The model under review builds one solid part; all positions refer to its coordinate system, in mm. A direction names the side the tool comes from. Give positions to 0.01 mm unless a question says otherwise; leave off trailing zeros. Order: outer loops, then holes, each group sorted by start corner. A loop starts at its lowest first (then second) coordinate and runs counter-clockwise, first axis right, second up. Notation, with made-up numbers: (-36, -13.5) - (8, -13.5) arc R25 cw to (8, -1.5) - close; hole circle Ø5 at (58.5, 82). An arc over 180 degrees is marked (long way). Use a Markdown table: item, result. Add a question column.
```python
from build123d import *

# Parameters (mm, degrees)
SKETCH2_R               = 1.651
BOSS_EXTRUDE1_DEPTH     = 68.58
CUT_EXTRUDE3_DEPTH      = 79.441187854
CUT_EXTRUDE3_DEPTH_BACK = 79.441187854
SKETCH3_R               = 3


with BuildPart() as part:
    # Sketch2 → Boss-Extrude1 (new body)
    with BuildSketch(Plane(origin=(0, 0, 0), x_dir=(0, 0, -1), z_dir=(1, 0, 0))):
        with BuildLine():
            Line((-12.7, 12.7), (12.7, 12.7))
            Line((12.7, 12.7), (12.7, 0))
            Line((12.7, 0), (26.924, 0))
            ThreePointArc((26.924, 0), (0, 26.924), (-26.924, 0))
            Line((-26.924, 0), (-12.7, 0))
            Line((-12.7, 0), (-12.7, 12.7))
        make_face()
        with Locations((14.368409794, 14.368409794)):
            Circle(SKETCH2_R, mode=Mode.SUBTRACT)
        with Locations((-14.368409794, 14.368409794)):
            Circle(SKETCH2_R, mode=Mode.SUBTRACT)
    extrude(amount=BOSS_EXTRUDE1_DEPTH)

    # Sketch3 → Cut-Extrude3 (cut, two sides: drawn at the far end of the back side and taken through both)
    with BuildSketch(Plane(origin=(0, 0, 0), x_dir=(1, 0, 0), z_dir=(0, 1, 0)).offset(-CUT_EXTRUDE3_DEPTH_BACK)):
        with Locations(Location((34.57387325, 0, 0), (0, 0, 180))):
            Circle(SKETCH3_R)
    extrude(amount=CUT_EXTRUDE3_DEPTH + CUT_EXTRUDE3_DEPTH_BACK, mode=Mode.SUBTRACT)


solid = part.part
```
Q1. We need section D-D (x = 22). Write out the cut boundary in (y, z).
Q2. We need section B-B (y = 7). Write out the cut boundary in (x, z), plus the area to 3 significant figures.
Q3. Clearance check with flat-ended pins moving along their axes: P1, Ø5.5, axis at x = 34.57, z = 0, coming from the -Y side; P2, Ø4, axis at x = 12.5, y = 23.5, coming from the -Z side; P3, Ø1, axis at x = 28.5, y = 17.5, coming from the +Z side; P4, Ø10, axis at x = 40, y = 8, coming from the -Z side. State where each tip first meets the part, or that it passes through.
Q4. Draft analysis for pull direction Z (two halves, no side actions). For faces 3 (the cylindrical face through (33.81, 16.005, 14.583)), 4 (the cylindrical face through (33.81, 25.497, 8.65)), 5 (the flat face through (0, 14, 0)), state which applies: pulls with the +Z half, pulls with the -Z half, needs draft (parallel to the pull), parting line crosses it, or undercut.
Q5. Machinability: for faces 1 (the cylindrical face through (33.81, 15.76, -15.26)), 2 (the flat face through (34, 12.7, 6)), which of the approach directions +Z, -Z, +X, -X, +Y, -Y give a long, thin tool a straight path to every point of the face, cutting with its end or side? Answer none if there is none.
Q6. We need section A-A (z = 0). Write out the cut boundary in (x, y), plus the area to 3 significant figures.
Q7. We need section C-C (y = 20.25). Write out the cut boundary in (x, z), plus the area to 3 significant figures.
Q8. Wall thickness on probe 1 along Z at (x, y) = (36, 1); probe 2 along Y at (x, z) = (4.5, 0); probe 3 along Z at (x, y) = (42, 3.25): over which ranges is each line inside the solid? List them lowest first.
Here are the results:
| question | item | result |
|---|---|---|
| 1 | outline | (0, -26.92) arc R26.92 ccw to (0, 26.92) - (0, 12.7) - (12.7, 12.7) - (12.7, -12.7) - (0, -12.7) - close; hole circle Ø3.3 at (14.37, -14.37); hole circle Ø3.3 at (14.37, 14.37) |
| 2 | outline | (0, -26) - (68.58, -26) - (68.58, -12.7) - (0, -12.7) - close; (0, 12.7) - (68.58, 12.7) - (68.58, 26) - (0, 26) - close |
| 2 | area | 1,820 mm2 |
| 3 | P1 | through |
| 3 | P2 | z = -16.21 |
| 3 | P3 | z = 20.88 |
| 3 | P4 | z = -26.76 |
| 4 | face 3 | undercut |
| 4 | face 4 | parting line crosses it |
| 4 | face 5 | needs draft |
| 5 | face 1 | +X, -X |
| 5 | face 2 | +X, -X, -Y |
| 6 | outline | (0, 12.7) - (31.57, 12.7) - (31.57, 26.92) - (0, 26.92) - close; (37.57, 12.7) - (68.58, 12.7) - (68.58, 26.92) - (37.57, 26.92) - close |
| 6 | area | 890 mm2 |
| 7 | outline | (0, -17.74) - (68.58, -17.74) - (68.58, 17.74) - (0, 17.74) - close; hole circle Ø6 at (34.57, 0) |
| 7 | area | 2,410 mm2 |
| 8 | probe 1 | -26.91 to -12.7, 12.7 to 26.91 |
| 8 | probe 2 | 12.7 to 26.92 |
| 8 | probe 3 | -26.73 to -12.7, 12.7 to 26.73 |
